For this review, use the dimensioned drawing (mm, ordinates from the lowest corner) and the shaded views. Give positions to 0.01 mm unless a question says otherwise; leave off trailing zeros. Loops run counter-clockwise (first coordinate to the right, second up) from the corner with the lowest first, then second, coordinate; pieces in that order, holes last. Notation, with made-up numbers: M -21.5,44.25 L 16.5,44.25 A26 cw 16.5,81.25 Z; hole C 25.5,-8 d7. An arc over 180 degrees is marked long. Use CSV: the item, a comma, the result in double quotes. Start each with the question number.
1. Take a section at C-C, the plane z = 3. Write out the cut boundary in (x, y), and give its area (3 significant figures).
2. Take a section at B-B, the plane y = 7.5. Write out the cut boundary in (x, z), and give its area (3 significant figures).
3. To check wall thickness, follow line 1 (Z direction, x = 2.75, y = 7.5); line 2 (Y direction, x = 1.6, z = 3); line 3 (Z direction, x = 3.7, y = 6.5). State the ranges of each line that lie inside material, in increasing order. Write a range as [from, to].
4. Take a section at D-D, the plane z = 12. Write out the cut boundary in (x, y), and give its area (3 significant figures).
5. Take a section at A-A, the plane x = 3.95. Write out the cut boundary in (y, z), and give its area (3 significant figures).
6. Insertion check: P1, Ø5, axis at y = 7.5, z = 3, coming from the -X side. The pin has a flat end and moves straight along its axis. Give the tip position at first contact, or say it passes through.
7. The part is to be moulded in two halves that separate along Y. For the marked faces 1, 2 and 3, say which applies: pulls with the +Y half, pulls with the -Y half, needs draft (parallel to the pull), parting line crosses it, or undercut.
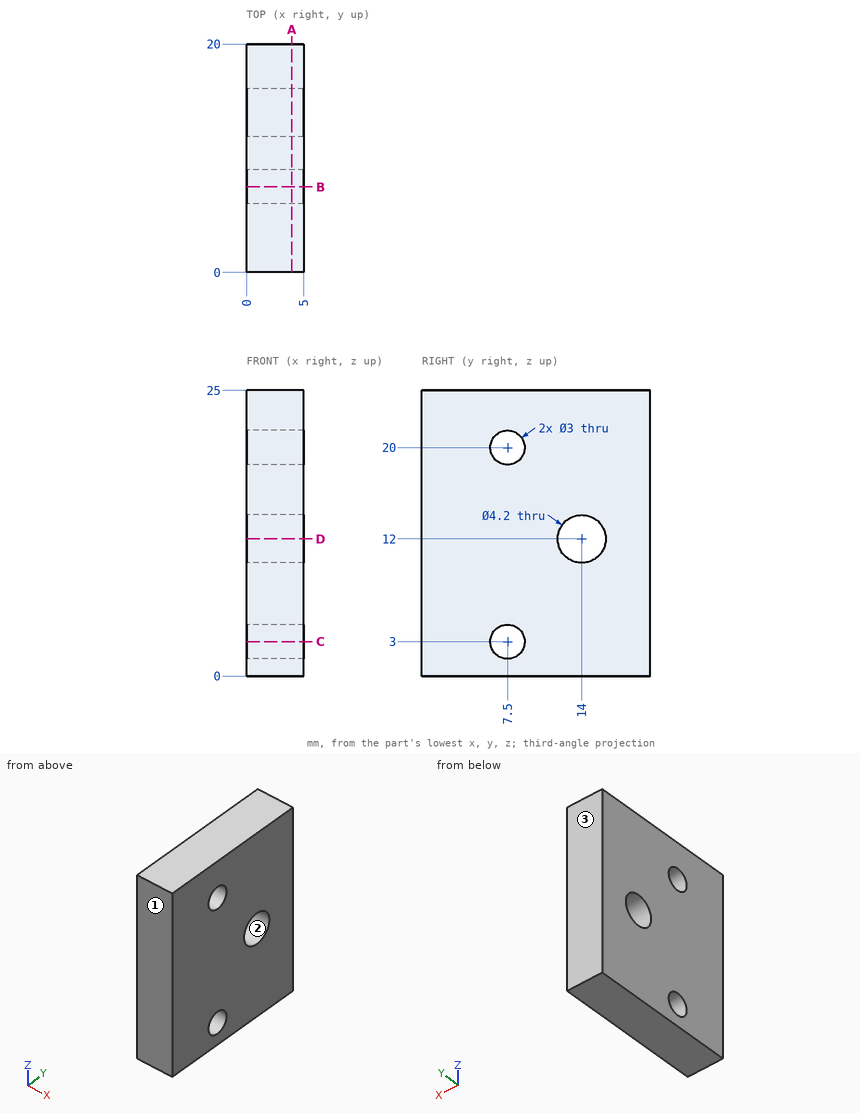
Result set:
1,outline,"M 0,0 L 5,0 L 5,6 L 0,6 Z; M 0,9 L 5,9 L 5,20 L 0,20 Z"
1,area,"85.0 mm2"
2,outline,"M 0,0 L 5,0 L 5,1.5 L 0,1.5 Z; M 0,4.5 L 5,4.5 L 5,18.5 L 0,18.5 Z; M 0,21.5 L 5,21.5 L 5,25 L 0,25 Z"
2,area,"95.0 mm2"
3,line 1,"[0, 1.5], [4.5, 18.5], [21.5, 25]"
3,line 2,"[0, 6], [9, 20]"
3,line 3,"[0, 1.88], [4.12, 18.88], [21.12, 25]"
4,outline,"M 0,0 L 5,0 L 5,11.9 L 0,11.9 Z; M 0,16.1 L 5,16.1 L 5,20 L 0,20 Z"
4,area,"79.0 mm2"
5,outline,"M 0,0 L 20,0 L 20,25 L 0,25 Z; hole C 7.5,3 d3; hole C 7.5,20 d3; hole C 14,12 d4.2"
5,area,"472 mm2"
6,P1,"x = 0"
7,face 1,"pulls with the -Y half"
7,face 2,"undercut"
7,face 3,"pulls with the +Y half"
